Can you work these out from the model? Positions are in its coordinate system, mm. Face numbers are marked on the shaded views. A direction names the side the tool comes from. Give positions to 0.01 mm unless a question says otherwise; leave off trailing zeros. Order: outer loops, then holes, each group sorted by start corner. A loop starts at its lowest first (then second) coordinate and runs counter-clockwise, first axis right, second up.
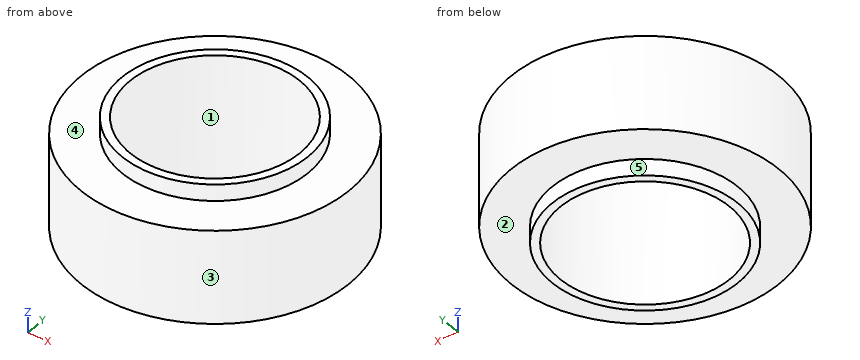
```python
from build123d import *

# Parameters (mm, degrees)
SCHIZZO1_R        = 49
SCHIZZO1_R_2      = 31
ESTRUSIONE1_DEPTH = 23
SCHIZZO4_W        = 15
SCHIZZO4_H        = 6


with BuildPart() as part:
    # Schizzo1 → Estrusione1 (new, symmetric)
    with BuildSketch(Plane.XY):
        Circle(SCHIZZO1_R)
        Circle(SCHIZZO1_R_2, mode=Mode.SUBTRACT)
    extrude(amount=ESTRUSIONE1_DEPTH, both=True)

    # Schizzo4 → Taglia-Rivoluzione1 (revolve, cut)
    with BuildSketch(Plane(origin=(0, 0, 0), x_dir=(1, 0, 0), z_dir=(0, 1, 0))):
        with Locations((41.5, 20)):
            Rectangle(SCHIZZO4_W, SCHIZZO4_H)
        with Locations((41.5, -20)):
            Rectangle(SCHIZZO4_W, SCHIZZO4_H)
    revolve(axis=Axis((0, 0, 23), (0, 0, -1)), mode=Mode.SUBTRACT)


solid = part.part
```
1) I'm going to push flat-ended pins straight in: pin 1 Ø4 at (x, z) = (19.5, 4) entering from -Y; pin 2 Ø6 at (y, z) = (13.5, 15) entering from +X; pin 3 Ø4 at (x, z) = (3.5, -6.5) entering from +Y. Where does each tip first touch, or does it pass through?
2) If I drill on line 1 (Y direction, x = 0.5, z = -20); line 2 (Y direction, x = 0, z = 4); line 3 (X direction, y = 1, z = -14), over which ranges is the centre line in solid material (lowest first)?
3) We'd pull the mould along Y, two halves only. Please class the marked faces 1, 2 and 3: +Y half, -Y half, draft (parallel to the pull), parting line (faces both ways), or undercut.
4) Which directions (+Z, -Z, +X, -X, +Y, -Y) give clear straight access to the entire face, cutting with the end or side of a thin tool? Please do the marked faces 4 and 5.
5) Suppose I cut it at C-C (z = -20). Please give me the cut outline in (x, y), and give its area (3 significant figures).
6) Suppose I cut it at A-A (x = 0). Please give me the cut outline in (y, z).
7) Suppose I cut it at D-D (x = 32.5). Please give me the cut outline in (y, z), and give its area (3 significant figures).
Results:
1. pin 1: stops at y = -45.77
1. pin 2: stops at x = 47.86
1. pin 3: stops at y = 48.98
2. line 1: y = -34 to -31, 31 to 34
2. line 2: y = -49 to -31, 31 to 49
2. line 3: x = -48.99 to -30.98, 30.98 to 48.99
3. face 1: undercut
3. face 2: draft
3. face 3: parting line
4. face 4: +Z
4. face 5: -Z
5. outline: circle Ø68 at (0, 0); hole circle Ø62 at (0, 0)
5. area: 613 mm2
6. outline: (-49, -17) - (-34, -17) - (-34, -23) - (-31, -23) - (-31, 23) - (-34, 23) - (-34, 17) - (-49, 17) - close; (31, -23) - (34, -23) - (34, -17) - (49, -17) - (49, 17) - (34, 17) - (34, 23) - (31, 23) - close
7. outline: (-36.67, -17) - (-9.99, -17) - (-9.99, -23) - (9.99, -23) - (9.99, -17) - (36.67, -17) - (36.67, 17) - (9.99, 17) - (9.99, 23) - (-9.99, 23) - (-9.99, 17) - (-36.67, 17) - close
7. area: 2,730 mm2
